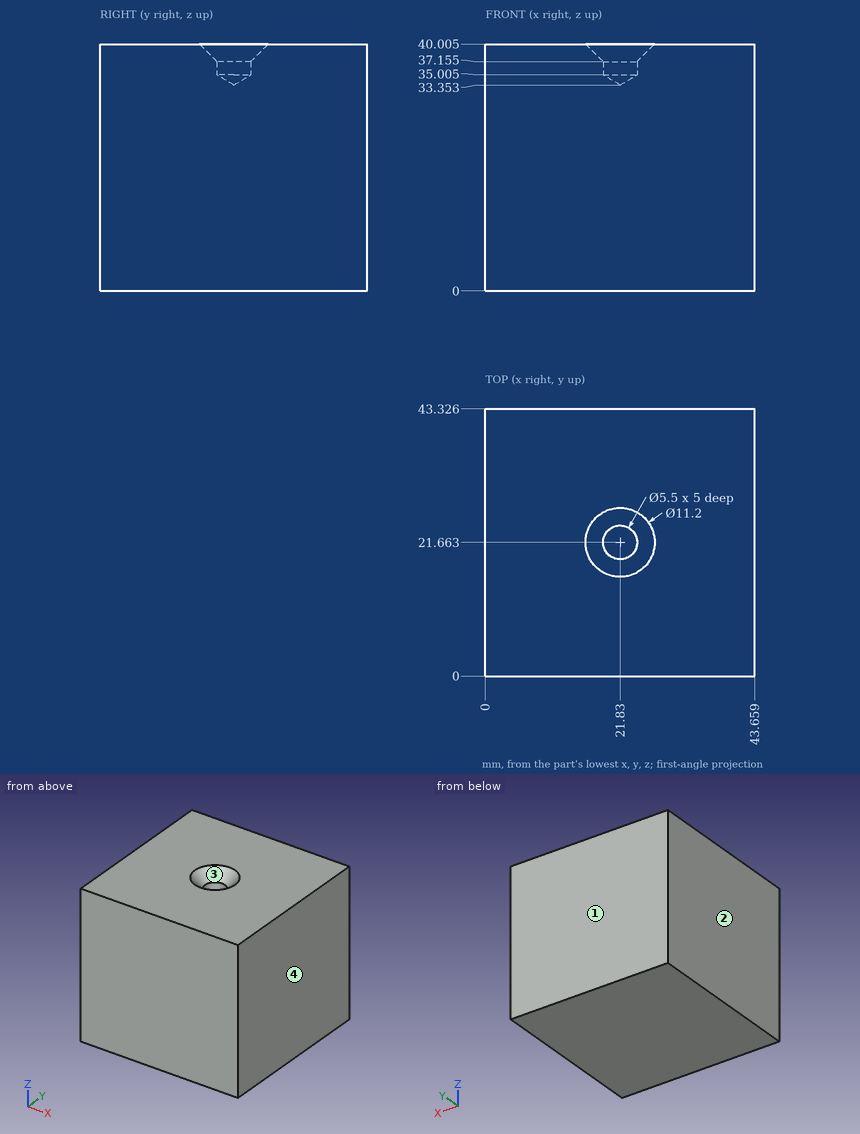
For this review, use the dimensioned drawing (mm, ordinates from the lowest corner) and the shaded views. Give positions to 0.01 mm unless a question says otherwise; leave off trailing zeros.
Item 1: Insertion check: pin 1 (12 mm diameter, centred on x = 27, z = 32, fed in from -Y). The pin has a flat end and moves straight along its axis. Give the tip position at first contact, or say it passes through.
Item 2: For line 1 along Z through (x, y) = (23.5, 22) (1 decimal), list the stretches that pass through material, from the lowest coordinate up.
Item 3: Draft analysis for pull direction X (two halves, no side actions). For the marked faces 1, 2, 3 and 4, state which applies: +X half, -X half, draft (parallel to the pull), parting line (faces both ways), or undercut.
Calculated:
1. pin 1: stops at y = 0
2. line 1: z = 0 to 34.4
3. face 1: draft
3. face 2: -X half
3. face 3: undercut
3. face 4: +X half
